Geometry: final body of the model. Coordinates: model frame, mm. Face numbers are marked on the shaded views. A direction names the side the tool comes from. Give positions to 0.01 mm unless a question says otherwise; leave off trailing zeros. Write each loop counter-clockwise with the first axis right and the second up, starting at its lowest first coordinate (ties: lowest second). Pieces come first, ordered by that corner, then holes. Notation, with made-up numbers: M 68.25,38.5 L 117.25,38.5 A16 cw 117.25,49.5 Z; hole C 20.25,14.5 d10. An arc over 180 degrees is marked long. Use one line per item in the form item = value. Start each with the question number.
Item 1: Contact query for flat-ended pins moving along their axis: P1, Ø3, axis at x = 2, y = 8.5, coming from the +Z side; P2, Ø1.5, axis at y = 8.5, z = 5.5, coming from the -X side; P3, Ø0.5, axis at x = 5, z = 5, coming from the -Y side. Output: stop coordinate, or through.
Item 2: Material intervals for line 1 along X through (y, z) = (11.75, 4.75); line 2 along Y through (x, z) = (-0.25, 2.25); line 3 along Z through (x, y) = (0.5, 2), sorted ascending. Write a range as from..to.
Item 3: Section query B-B on x = 2.25. Return loops of the section in (y, z), then the cut area to 3 significant figures.
Item 4: Section query D-D on y = 8.75. Return loops of the section in (x, z).
Item 5: Section query A-A on z = 6.75. Return loops of the section in (x, y), then the cut area to 3 significant figures.
Item 6: Access query for the marked faces 5, 6 and 7. Directions: +Z, -Z, +X, -X, +Y, -Y. A direction counts if a zero-diameter tool reaches every point of the face in a straight line with its end or side. Return the directions, or none.
Item 7: Pull-direction query (X, two-part tool) for the marked faces 1, 2, 3 and 4; classes: released by +X, released by -X, zero draft, split by the parting line, or undercut.
Item 8: Section query C-C on z = 0.5. Return loops of the section in (x, y), then the cut area to 3 significant figures.
from build123d import *

# Parameters (mm, degrees)
SKETCH1_W           = 7
SKETCH1_H           = 9.5
BOSS_EXTRUDE1_DEPTH = 12
SKETCH3_R           = 3.15
CUT_EXTRUDE2_DEPTH  = 11
SKETCH4_W           = 1
SKETCH4_H           = 2
BOSS_EXTRUDE2_DEPTH = 4


with BuildPart() as part:
    # Sketch1 → Boss-Extrude1 (new body)
    with BuildSketch(Plane(origin=(0, 0, 0), x_dir=(1, 0, 0), z_dir=(0, 1, 0))):
        with Locations((1.651810585, 0.915738162)):
            Rectangle(SKETCH1_W, SKETCH1_H)
    extrude(amount=BOSS_EXTRUDE1_DEPTH)

    # Sketch3 → Cut-Extrude2 (cut)
    with BuildSketch(Plane.XZ):
        with Locations(Location((1.651810585, -0.165738162, 0), (0, 0, 270))):
            Circle(SKETCH3_R)
    extrude(amount=-CUT_EXTRUDE2_DEPTH, mode=Mode.SUBTRACT)

    # Sketch4 → Boss-Extrude2 (add)
    with BuildSketch(Plane.XY.offset(3.834261838)):
        with Locations((-1.348189415, 11)):
            Rectangle(SKETCH4_W, SKETCH4_H)
        with Locations((4.651810585, 11)):
            Rectangle(SKETCH4_W, SKETCH4_H)
    extrude(amount=BOSS_EXTRUDE2_DEPTH)


solid = part.part
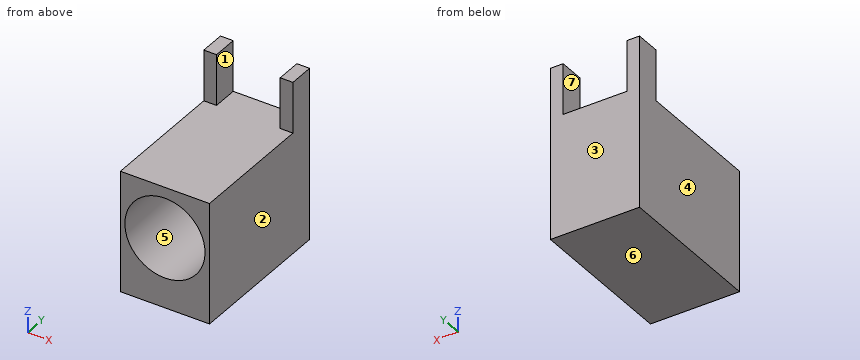
Answer sheet:
q1.P1 = 3.83
q1.P2 = through
q1.P3 = 10
q2.line_1 = -1.85..-0.85, 4.15..5.15
q2.line_2 = 11..12
q2.line_3 = -5.67..-3.1, 2.77..3.83
q3.outline = M 0,-5.67 L 12,-5.67 L 12,3.83 L 0,3.83 L 0,2.93 L 11,2.93 L 11,-3.26 L 0,-3.26 Z
q3.area = 46.0 mm2
q4.outline = M -1.85,-5.67 L 5.15,-5.67 L 5.15,3.83 L -1.85,3.83 Z; hole C 1.65,-0.17 d6.3
q5.outline = M -1.85,10 L -0.85,10 L -0.85,12 L -1.85,12 Z; M 4.15,10 L 5.15,10 L 5.15,12 L 4.15,12 Z
q5.area = 4.00 mm2
q6.face_5 = -Y
q6.face_6 = -Z, +X, -X, +Y, -Y
q6.face_7 = +Z, +Y, -Y
q7.face_1 = undercut
q7.face_2 = released by +X
q7.face_3 = zero draft
q7.face_4 = released by -X
q8.outline = M -1.85,0 L -1.43,0 L -1.43,11 L 4.73,11 L 4.73,0 L 5.15,0 L 5.15,12 L -1.85,12 Z
q8.area = 16.3 mm2
